Read the model definition and answer for the solid it produces. Units are mm, in the model's axes. A direction names the side the tool comes from. Coordinates: 2 decimals unless noted, no trailing zeros. Order: outer loops, then holes, each group sorted by start corner. A loop starts at its lowest first (then second) coordinate and runs counter-clockwise, first axis right, second up. Notation, with made-up numbers: (0, 67) -> (40, 67) arc R23 ccw to (40, 90) -> close; hole circle Ø1 at (39.5, 5.25). An arc over 180 degrees is marked (long way). Answer as a JSON object with one key per item and string values. Group by question number.
1) Consider L1, parallel to Y at x = 32.5, z = -0.75; L2, parallel to X at y = 5.75, z = -36.5; L3, parallel to Z at x = 35.5, y = 17.5. Determine where each line is inside the solid, lowest interval first.
2) Section C-C on y = 5.5 is taken. Determine the outline of the cut face in (x, z), and give its area (3 significant figures).
3) Section A-A on y = 17.5 is taken. Determine the outline of the cut face in (x, z), and give its area (3 significant figures).
4) Determine the mould class of faces 1 (the flat face through (19, 10, 0)), 2 (the flat face through (37, 9.2, -9.5)), 3 (the cylindrical face through (19.39, 18.51, -0.49)) for opening direction X: released by +X, released by -X, zero draft, split by the parting line, or undercut.
5) Given pin 1 (9 mm diameter, centred on y = 6, z = -23.5, fed in from +X); pin 2 (4 mm diameter, centred on y = 7, z = -6, fed in from +X); pin 3 (5 mm diameter, centred on x = 20.5, y = 2.5, fed in from -Z), each flat-ended and moving along its own axis, determine where each tip first touches the part or whether it passes through.
6) Section D-D on z = -15 is taken. Determine the outline of the cut face in (x, y), and give its area (3 significant figures).
7) Section B-B on x = 15 is taken. Determine the outline of the cut face in (y, z).
8) A tool of negligible diameter and unlimited length cuts with its end or side. For faces 4 (the cylindrical face through (31, 2.57, -0.49)), 5 (the flat face through (23, 10, -9)), 6 (the flat face through (23, 10, -10)), from which of +Z, -Z, +X, -X, +Y, -Y can it reach the whole face along a straight path? Write none if from no direction.
from build123d import *
from build123d.topology import SkipClean

# Parameters (mm, degrees)
EXTRUDE_1_DEPTH     = 20
MM_PRESS_1_D        = 3
SKETCH_4_W          = 8
SKETCH_4_H          = 18
CUT_EXTRUDE_1_DEPTH = 34
SKETCH_5_W          = 8
SKETCH_5_H          = 18
CUT_EXTRUDE_3_DEPTH = 36
SKETCH_7_W          = 10
SKETCH_7_H          = 20
SKETCH_7_W_2        = 8
SKETCH_7_H_2        = 18
EXTRUDE_2_DEPTH     = 14


with BuildPart() as part:
    # 草图1 → 凸台-拉伸1 (new body)
    with BuildSketch(Plane(origin=(0, 0, 0), x_dir=(1, 0, 0), z_dir=(0, 1, 0))):
        Polygon((0, 0), (0, 35), (10, 35), (10, 10), (37, 10), (37, 0), align=None)
    extrude(amount=EXTRUDE_1_DEPTH)

    # 大小mm Press 暗销孔1 (through all)
    with Locations(Plane(origin=(20.5, 2.5, -10), x_dir=(-1, 0, 0), z_dir=(0, 0, -1))):
        with Locations((0, 0), (-12, 0), (-12, 15), (0, 15)):
            Hole(MM_PRESS_1_D / 2)

    # 草图4 → 切除-拉伸1 (cut)
    with BuildSketch(Plane(origin=(0, 0, -35), x_dir=(-1, 0, 0), z_dir=(0, 0, -1))):
        with Locations((-5, 10)):
            Rectangle(SKETCH_4_W, SKETCH_4_H)
    extrude(amount=-CUT_EXTRUDE_1_DEPTH, mode=Mode.SUBTRACT)

    # 草图5 → 切除-拉伸3 (cut)
    with SkipClean():  # the faces are left unmerged after this step: merging them gives an invalid solid
        with BuildSketch(Plane(origin=(37, 0, 0), x_dir=(0, 0, -1), z_dir=(1, 0, 0))):
            with Locations((5, 10)):
                Rectangle(SKETCH_5_W, SKETCH_5_H)
        extrude(amount=-CUT_EXTRUDE_3_DEPTH, mode=Mode.SUBTRACT)

    # 草图7 → 凸台-拉伸2 (add)
    with SkipClean():  # the faces are left unmerged after this step: merging them gives an invalid solid
        with BuildSketch(Plane(origin=(0, 0, -35), x_dir=(-1, 0, 0), z_dir=(0, 0, -1))):
            with Locations((-5, 10)):
                Rectangle(SKETCH_7_W, SKETCH_7_H)
            with Locations((-5, 10)):
                Rectangle(SKETCH_7_W_2, SKETCH_7_H_2, mode=Mode.SUBTRACT)
        extrude(amount=EXTRUDE_2_DEPTH)


solid = part.part
Worked answers:
{
 "1": {"L1": "y = 0 to 1, 4 to 16, 19 to 20", "L2": "x = 0 to 1, 9 to 10", "L3": "z = -10 to -9, -1 to 0"},
 "2": {"outline": "(0, -49) -> (1, -49) -> (1, -1) -> (37, -1) -> (37, 0) -> (0, 0) -> close; (9, -49) -> (10, -49) -> (10, -10) -> (37, -10) -> (37, -9) -> (9, -9) -> close", "area": "152 mm²"},
 "3": {"outline": "(0, -49) -> (1, -49) -> (1, -1) -> (19, -1) -> (19, 0) -> (0, 0) -> close; (9, -49) -> (10, -49) -> (10, -10) -> (19, -10) -> (19, -9) -> (9, -9) -> close; (22, -10) -> (31, -10) -> (31, -9) -> (22, -9) -> close; (22, -1) -> (31, -1) -> (31, 0) -> (22, 0) -> close; (34, -10) -> (37, -10) -> (37, -9) -> (34, -9) -> close; (34, -1) -> (37, -1) -> (37, 0) -> (34, 0) -> close", "area": "140 mm²"},
 "4": {"face 1": "zero draft", "face 2": "released by +X", "face 3": "undercut"},
 "5": {"pin 1": "stops at x = 10", "pin 2": "stops at x = 1", "pin 3": "stops at z = -10"},
 "6": {"outline": "(0, 0) -> (10, 0) -> (10, 20) -> (0, 20) -> close; hole (1, 1) -> (9, 1) -> (9, 19) -> (1, 19) -> close", "area": "56.0 mm²"},
 "7": {"outline": "(0, -10) -> (20, -10) -> (20, 0) -> (0, 0) -> close; hole (1, -9) -> (19, -9) -> (19, -1) -> (1, -1) -> close"},
 "8": {"face 4": "+Z, -Z", "face 5": "+X", "face 6": "-Z, +X, +Y, -Y"}
}
